from build123d import *

# Parameters (mm, degrees)
CYLINDER023_R     = 1.38
CYLINDER023_DEPTH = 30
CYLINDER022_R     = 1.38
CYLINDER022_DEPTH = 30
CYLINDER021_R     = 1.38
CYLINDER021_DEPTH = 30
CYLINDER020_R     = 1.38
CYLINDER020_DEPTH = 30
BOX006_W          = 10
BOX006_H          = 65
BOX006_DEPTH      = 35
BOX011_W          = 20
BOX011_H          = 35
BOX011_DEPTH      = 10
BOX010_W          = 29
BOX010_H          = 20
BOX010_DEPTH      = 10
BOX009_W          = 29
BOX009_H          = 20
BOX009_DEPTH      = 10
BOX008_W          = 44
BOX008_H          = 20
BOX008_DEPTH      = 10
BOX007_W          = 44
BOX007_H          = 20
BOX007_DEPTH      = 10
BOX005_W          = 114
BOX005_H          = 69
BOX005_DEPTH      = 35
BOX004_W          = 120
BOX004_H          = 75
BOX004_DEPTH      = 35


with BuildPart() as cylinder023:
    # Cylinder023 → Cylinder023 (new body)
    with BuildSketch(Plane(origin=(74, 61, -2), x_dir=(1, 0, 0), z_dir=(0, 0, 1))):
        Circle(CYLINDER023_R)
    extrude(amount=CYLINDER023_DEPTH)


with BuildPart() as cylinder022:
    # Cylinder022 → Cylinder022 (new body)
    with BuildSketch(Plane(origin=(16, 61, -2), x_dir=(1, 0, 0), z_dir=(0, 0, 1))):
        Circle(CYLINDER022_R)
    extrude(amount=CYLINDER022_DEPTH)


with BuildPart() as cylinder021:
    # Cylinder021 → Cylinder021 (new body)
    with BuildSketch(Plane(origin=(16, 12, -2), x_dir=(1, 0, 0), z_dir=(0, 0, 1))):
        Circle(CYLINDER021_R)
    extrude(amount=CYLINDER021_DEPTH)


with BuildPart() as fusion008:
    # Cylinder020 → Cylinder020 (new body)
    with BuildSketch(Plane(origin=(74, 12, -2), x_dir=(1, 0, 0), z_dir=(0, 0, 1))):
        Circle(CYLINDER020_R)
    extrude(amount=CYLINDER020_DEPTH)

    # Fusion008: union Cylinder023, Cylinder022, Cylinder021
    add(cylinder023.part)
    add(cylinder022.part)
    add(cylinder021.part)


with BuildPart() as kegel003:
    # Cone003 → Cone003 (revolve)
    with BuildSketch(Plane(origin=(16, 61, 3), x_dir=(1, 0, 0), z_dir=(0, -1, 0))):
        Polygon((0, 0), (4, 0), (2.9, 22), (0, 22), align=None)
    revolve(axis=Axis((16, 61, 3), (0, 0, 1)))


with BuildPart() as kegel002:
    # Cone002 → Cone002 (revolve)
    with BuildSketch(Plane(origin=(16, 12, 3), x_dir=(1, 0, 0), z_dir=(0, -1, 0))):
        Polygon((0, 0), (4, 0), (2.9, 22), (0, 22), align=None)
    revolve(axis=Axis((16, 12, 3), (0, 0, 1)))


with BuildPart() as kegel001:
    # Cone001 → Cone001 (revolve)
    with BuildSketch(Plane(origin=(74, 61, 3), x_dir=(1, 0, 0), z_dir=(0, -1, 0))):
        Polygon((0, 0), (4, 0), (2.9, 22), (0, 22), align=None)
    revolve(axis=Axis((74, 61, 3), (0, 0, 1)))


with BuildPart() as fusion015:
    # Cone → Cone (revolve)
    with BuildSketch(Plane(origin=(74, 12, 3), x_dir=(1, 0, 0), z_dir=(0, -1, 0))):
        Polygon((0, 0), (4, 0), (2.9, 22), (0, 22), align=None)
    revolve(axis=Axis((74, 12, 3), (0, 0, 1)))

    # Fusion015: union Kegel003, Kegel002, Kegel001
    add(kegel003.part)
    add(kegel002.part)
    add(kegel001.part)


with BuildPart() as obj1:
    # Box006 → Box006 (new body)
    with BuildSketch(Plane(origin=(115, 5, 5), x_dir=(1, 0, 0), z_dir=(0, 0, 1))):
        with Locations((5, 32.5)):
            Rectangle(BOX006_W, BOX006_H)
    extrude(amount=BOX006_DEPTH)


with BuildPart() as obj2:
    # Box011 → Box011 (new body)
    with BuildSketch(Plane(origin=(-10, 19, 26), x_dir=(1, 0, 0), z_dir=(0, 0, 1))):
        with Locations((10, 17.5)):
            Rectangle(BOX011_W, BOX011_H)
    extrude(amount=BOX011_DEPTH)


with BuildPart() as obj3:
    # Box010 → Box010 (new body)
    with BuildSketch(Plane(origin=(81, 60, 26), x_dir=(1, 0, 0), z_dir=(0, 0, 1))):
        with Locations((14.5, 10)):
            Rectangle(BOX010_W, BOX010_H)
    extrude(amount=BOX010_DEPTH)


with BuildPart() as obj4:
    # Box009 → Box009 (new body)
    with BuildSketch(Plane(origin=(81, -10, 26), x_dir=(1, 0, 0), z_dir=(0, 0, 1))):
        with Locations((14.5, 10)):
            Rectangle(BOX009_W, BOX009_H)
    extrude(amount=BOX009_DEPTH)


with BuildPart() as obj5:
    # Box008 → Box008 (new body)
    with BuildSketch(Plane(origin=(23, 68, 26), x_dir=(1, 0, 0), z_dir=(0, 0, 1))):
        with Locations((22, 10)):
            Rectangle(BOX008_W, BOX008_H)
    extrude(amount=BOX008_DEPTH)


with BuildPart() as fusion014:
    # Box007 → Box007 (new body)
    with BuildSketch(Plane(origin=(23, -10, 26), x_dir=(1, 0, 0), z_dir=(0, 0, 1))):
        with Locations((22, 10)):
            Rectangle(BOX007_W, BOX007_H)
    extrude(amount=BOX007_DEPTH)

    # Fusion010: union obj2, obj3, obj4, obj5
    add(obj2.part)
    add(obj3.part)
    add(obj4.part)
    add(obj5.part)

    # Fusion014: union obj1
    add(obj1.part)


with BuildPart() as obj6:
    # Box005 → Box005 (new body)
    with BuildSketch(Plane(origin=(3, 3, 3), x_dir=(1, 0, 0), z_dir=(0, 0, 1))):
        with Locations((57, 34.5)):
            Rectangle(BOX005_W, BOX005_H)
    extrude(amount=BOX005_DEPTH)


with BuildPart() as obj7:
    # Box004 → Box004 (new body)
    with BuildSketch(Plane.XY):
        with Locations((60, 37.5)):
            Rectangle(BOX004_W, BOX004_H)
    extrude(amount=BOX004_DEPTH)

    # Cut006: cut obj6
    add(obj6.part, mode=Mode.SUBTRACT)

    # Cut007: cut Fusion014
    add(fusion014.part, mode=Mode.SUBTRACT)

    # Fusion016: union Fusion015
    add(fusion015.part)

    # Cut008: cut Fusion008
    add(fusion008.part, mode=Mode.SUBTRACT)


solid = obj7.part
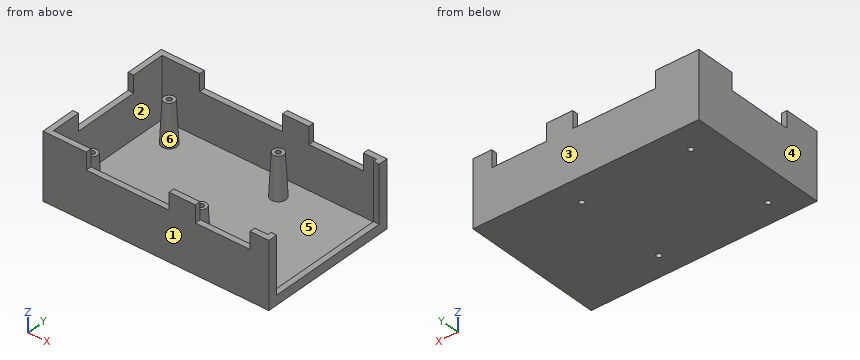
Could you check a few things on this model? Use its own coordinates, in mm. Face numbers are marked on the shaded views. A direction names the side the tool comes from. Round coordinates to 2 decimals unless told otherwise and drop trailing zeros. Order: outer loops, then holes, each group sorted by start corner. A loop starts at its lowest first (then second) coordinate and runs counter-clockwise, first axis right, second up.
Q1. Imagine slicing it at B-B, the plane z = 30.5. State how many separate pieces and enclosed holes the cut face has, then the cut area to 3 significant figures.
Geometry says:
separate pieces: 6
enclosed holes: 0
area: 396 mm2
Q2. I'm going to push flat-ended pins straight in: P1, Ø12, axis at x = 106, y = 51, coming from the +Z side; P2, Ø0.9, axis at x = 99, y = 1.5, coming from the +Z side; P3, Ø4.5, axis at x = 74, y = 61, coming from the +Z side. Where does each tip first touch, or does it pass through?
Geometry says:
P1: stops at z = 3
P2: stops at z = 26
P3: stops at z = 25
Q3. Imagine slicing it at D-D, the plane x = 74. List the corners of the cut face in (y, z) for me, then the cut area to 3 significant figures.
Geometry says:
outline: (0, 0) - (10.62, 0) - (10.62, 25) - (9.1, 25) - (8, 3) - (3, 3) - (3, 35) - (0, 35) - close; (13.38, 0) - (59.62, 0) - (59.62, 25) - (58.1, 25) - (57, 3) - (16, 3) - (14.9, 25) - (13.38, 25) - close; (62.38, 0) - (75, 0) - (75, 35) - (72, 35) - (72, 3) - (65, 3) - (63.9, 25) - (62.38, 25) - close
area: 583 mm2
Q4. Please list where these lines run through material, in increasing order: probe 1 along Y at (x, z) = (76, 17.5); probe 2 along Y at (x, z) = (25, 12); probe 3 along Z at (x, y) = (42.5, 57.5).
Geometry says:
probe 1: y = 0 to 3, 9.41 to 14.59, 58.41 to 63.59, 72 to 75
probe 2: y = 0 to 3, 72 to 75
probe 3: z = 0 to 3
Q5. Imagine slicing it at A-A, the plane y = 61. List the corners of the cut face in (x, z) for me.
Geometry says:
outline: (0, 0) - (14.62, 0) - (14.62, 25) - (13.1, 25) - (12, 3) - (3, 3) - (3, 35) - (0, 35) - close; (17.38, 0) - (72.62, 0) - (72.62, 25) - (71.1, 25) - (70, 3) - (20, 3) - (18.9, 25) - (17.38, 25) - close; (75.38, 0) - (120, 0) - (120, 5) - (117, 5) - (117, 3) - (78, 3) - (76.9, 25) - (75.38, 25) - close
Q6. Thinking about a two-plate mould opening in X: for the marked faces 3, 4, 5 and 6, which applies, released by +X, released by -X, zero draft, split by the parting line, or undercut?
Geometry says:
face 3: zero draft
face 4: released by -X
face 5: undercut
face 6: undercut
Q7. Which directions (+Z, -Z, +X, -X, +Y, -Y) give clear straight access to the entire face, cutting with the end or side of a thin tool? Please do the marked faces 1 and 2.
Geometry says:
face 1: +Z, -Z, +X, -X, -Y
face 2: +Z
Q8. Imagine slicing it at C-C, the plane x = 101. List the corners of the cut face in (y, z) for me, then the cut area to 3 significant figures.
Geometry says:
outline: (0, 0) - (75, 0) - (75, 26) - (72, 26) - (72, 3) - (3, 3) - (3, 26) - (0, 26) - close
area: 363 mm2
